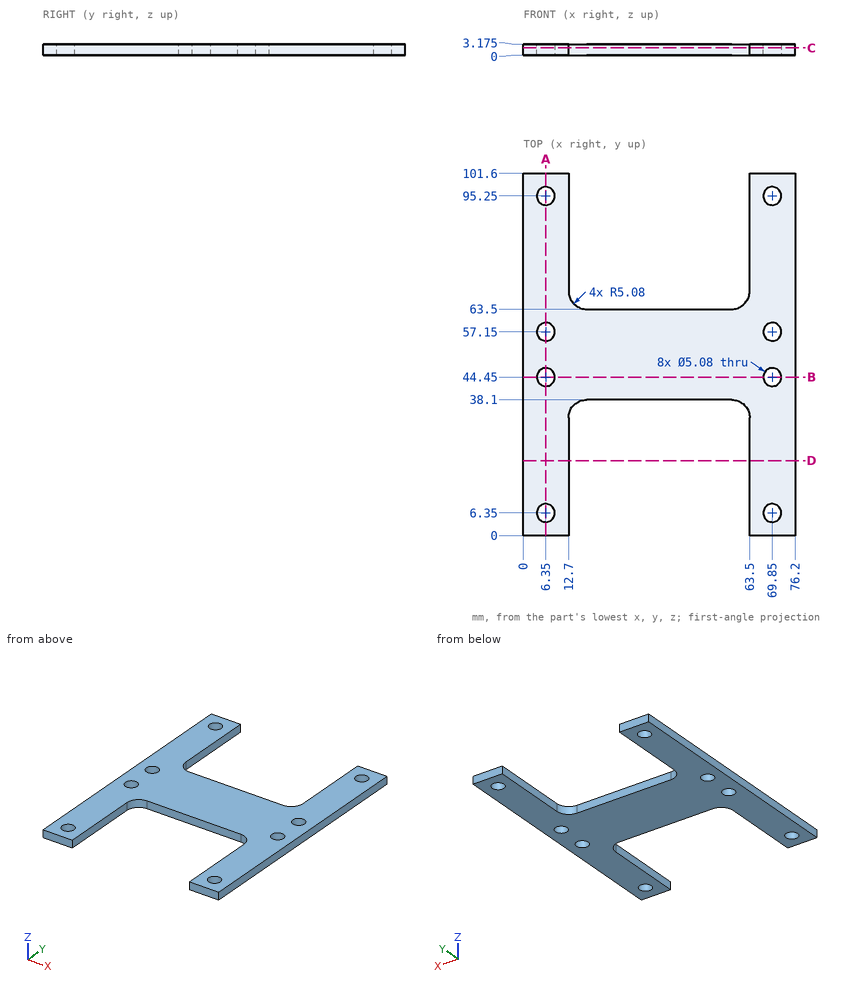
Design review of the part shown in the three views and the two pictorial views. Dimensions are in mm from the part's minimum x, y and z. Round coordinates to 2 decimals unless told otherwise and drop trailing zeros. Write each loop counter-clockwise with the first axis right and the second up, starting at its lowest first coordinate (ties: lowest second). Pieces come first, ordered by that corner, then holes.
Item 1: For probe 1 along Y at (x, z) = (6.35, 0.7); probe 2 along X at (y, z) = (95.25, 2.3); probe 3 along X at (y, z) = (79.5, 2.55), list the stretches that pass through material, from the lowest coordinate up.
Item 2: Clearance check with flat-ended pins moving along their axes: pin 1 Ø1.5 at (x, z) = (15.5, 1.5) entering from -Y; pin 2 Ø1 at (x, z) = (39, 2) entering from +Y; pin 3 Ø4 at (x, y) = (69.85, 95.25) entering from -Z. State where each tip first meets the part, or that it passes through.
Item 3: We need section A-A on x = 6.35. Write out the cut boundary in (y, z) (3 decimals).
Item 4: We need section D-D on y = 21. Write out the cut boundary in (x, z) (3 decimals).
Item 5: We need section B-B on y = 44.45. Write out the cut boundary in (x, z) (3 decimals), and give its area (3 significant figures).
Item 6: We need section C-C on z = 2.1. State how many separate pieces and enclosed holes the cut face has, and give its area (3 significant figures).
Returned:
1. probe 1: y = 0 to 3.81, 8.89 to 41.91, 46.99 to 54.61, 59.69 to 92.71, 97.79 to 101.6
1. probe 2: x = 0 to 3.81, 8.89 to 12.7, 63.5 to 67.31, 72.39 to 76.2
1. probe 3: x = 0 to 12.7, 63.5 to 76.2
2. pin 1: stops at y = 37.1
2. pin 2: stops at y = 63.5
2. pin 3: passes through
3. outline: (0, 0) - (3.81, 0) - (3.81, 3.175) - (0, 3.175) - close; (8.89, 0) - (41.91, 0) - (41.91, 3.175) - (8.89, 3.175) - close; (46.99, 0) - (54.61, 0) - (54.61, 3.175) - (46.99, 3.175) - close; (59.69, 0) - (92.71, 0) - (92.71, 3.175) - (59.69, 3.175) - close; (97.79, 0) - (101.6, 0) - (101.6, 3.175) - (97.79, 3.175) - close
4. outline: (0, 0) - (12.7, 0) - (12.7, 3.175) - (0, 3.175) - close; (63.5, 0) - (76.2, 0) - (76.2, 3.175) - (63.5, 3.175) - close
5. outline: (0, 0) - (3.81, 0) - (3.81, 3.175) - (0, 3.175) - close; (8.89, 0) - (67.31, 0) - (67.31, 3.175) - (8.89, 3.175) - close; (72.39, 0) - (76.2, 0) - (76.2, 3.175) - (72.39, 3.175) - close
5. area: 210 mm2
6. separate pieces: 1
6. enclosed holes: 8
6. area: 3,730 mm2
